Can you work these out from the model? Positions are in its coordinate system, mm. A direction names the side the tool comes from. Coordinates: 2 decimals unless noted, no trailing zeros. Write each loop counter-clockwise with the first axis right and the second up, starting at its lowest first coordinate (ties: lowest second). Pieces come first, ordered by that corner, then holes. Notation, with made-up numbers: (-5.75, 85.25) -> (11.25, 85.25) arc R20 ccw to (11.25, 104.25) -> close; hole circle Ø10 at (33.25, 3.25). An arc over 180 degrees is marked (long way). Use one line per item in the form item = value.
```python
from build123d import *

# Parameters (mm, degrees)
BOSS_EXTRUDE2_DEPTH       = 60
SKETCH4_W                 = 120
SKETCH4_H                 = 100
BOSS_EXTRUDE3_DEPTH       = 7.5
SKETCH5_W                 = 135
SKETCH5_H                 = 150
BOSS_EXTRUDE4_DEPTH       = 5
SKETCH6_W                 = 112.3
SKETCH6_H                 = 75
CUT_EXTRUDE2_DEPTH        = 75
F_10_CLEARANCE_HOLE1_D    = 4.7752
F_2_CLEARANCE_HOLE1_D     = 2.032
F_2_CLEARANCE_HOLE1_DEPTH = 6.35
F_2_CLEARANCE_HOLE1_TIP   = 0.610474389
SKETCH17_W                = 3
SKETCH17_H                = 3
CUT_EXTRUDE4_DEPTH        = 76
SKETCH18_R                = 2.5
CUT_EXTRUDE5_DEPTH        = 27
SKETCH19_R                = 1.5
CUT_EXTRUDE6_DEPTH        = 4


with BuildPart() as part:
    # Sketch3 → Boss-Extrude2 (new body, symmetric)
    with BuildSketch(Plane.XY):
        with BuildLine():
            Line((0, 0), (120, 0))
            Line((120, 0), (120, 100))
            Line((120, 100), (115, 100))
            ThreePointArc((115, 100), (54.85834395, 118.924191085), (0, 150))
            Line((0, 150), (0, 0))
        make_face()
    extrude(amount=BOSS_EXTRUDE2_DEPTH, both=True)

    # Sketch4 → Boss-Extrude3 (add)
    with BuildSketch(Plane.XY.offset(60)):
        with Locations((60, 50)):
            Rectangle(SKETCH4_W, SKETCH4_H)
    boss_extrude3 = extrude(amount=BOSS_EXTRUDE3_DEPTH)

    # Mirror1: Boss-Extrude3 across plane
    add(boss_extrude3.mirror(Plane.XY))

    # Sketch5 → Boss-Extrude4 (add)
    with BuildSketch(Plane.ZY):
        with Locations((0, 75)):
            Rectangle(SKETCH5_W, SKETCH5_H)
    extrude(amount=BOSS_EXTRUDE4_DEPTH)

    # Sketch6 → Cut-Extrude2 (cut)
    with BuildSketch(Plane.XZ):
        with Locations((51.15, 0)):
            Rectangle(SKETCH6_W, SKETCH6_H)
    extrude(amount=-CUT_EXTRUDE2_DEPTH, mode=Mode.SUBTRACT)

    # #10 Clearance Hole1 (through all)
    with Locations(Plane.ZY.offset(-107.3)):
        with Locations((0, 55), (0, 20)):
            Hole(F_10_CLEARANCE_HOLE1_D / 2)

    # #2 Clearance Hole1
    with Locations(Plane(origin=(0, 75, 0), x_dir=(-1, 0, 0), z_dir=(0, -1, 0))):
        with Locations((-20, 18.5), (-72, -14.25), (-72, 13.75), (-21.143, -29.5)):
            Hole(F_2_CLEARANCE_HOLE1_D / 2, depth=F_2_CLEARANCE_HOLE1_DEPTH)
            with Locations((0, 0, -(F_2_CLEARANCE_HOLE1_DEPTH + F_2_CLEARANCE_HOLE1_TIP / 2))):  # 118° drill point
                Cone(0, F_2_CLEARANCE_HOLE1_D / 2, F_2_CLEARANCE_HOLE1_TIP, mode=Mode.SUBTRACT)

    # Sketch15 → #10 Clearance Hole2 (revolve, cut)
    with BuildSketch(Plane(origin=(15, 115, 60), x_dir=(0, -1, 0), z_dir=(1, 0, 0))):
        Polygon((0, 0), (0, 26.849876674), (2.413, 25.4), (2.413, 0), align=None)
    f_10_clearance_hole2 = revolve(axis=Axis((15, 115, 66.35), (0, 0, -1)), mode=Mode.SUBTRACT)

    # Mirror2: #10 Clearance Hole2 across plane
    add(f_10_clearance_hole2.mirror(Plane.XY), mode=Mode.SUBTRACT)

    # Sketch17 → Cut-Extrude4 (cut, through all)
    with BuildSketch(Plane.XZ.offset(-75)):
        with Locations((4.5, 0)):
            Rectangle(SKETCH17_W, SKETCH17_H)
    extrude(amount=-CUT_EXTRUDE4_DEPTH, mode=Mode.SUBTRACT)

    # Sketch18 → Cut-Extrude5 (cut)
    with BuildSketch(Plane(origin=(0, 0, 37.5), x_dir=(-1, 0, 0), z_dir=(0, 0, -1))):
        with Locations((-67.5, 30)):
            Circle(SKETCH18_R)
        with Locations((-57.5, 30)):
            Circle(SKETCH18_R)
        with Locations((-47.5, 30)):
            Circle(SKETCH18_R)
    extrude(amount=-CUT_EXTRUDE5_DEPTH, mode=Mode.SUBTRACT)

    # Sketch19 → Cut-Extrude6 (cut, through all)
    with BuildSketch(Plane(origin=(0, 0, 64.5), x_dir=(-1, 0, 0), z_dir=(0, 0, -1))):
        with Locations((-67.5, 30)):
            Circle(SKETCH19_R)
        with Locations((-57.5, 30)):
            Circle(SKETCH19_R)
        with Locations((-47.5, 30)):
            Circle(SKETCH19_R)
    extrude(amount=-CUT_EXTRUDE6_DEPTH, mode=Mode.SUBTRACT)


solid = part.part
```
Q1. Suppose I cut it at B-B (z = -50). Write out the boundary of the cut face in (x, y).
Return value:
outline = (-5, 0) -> (120, 0) -> (120, 100) -> (115, 100) arc R300 cw to (0, 150) -> (-5, 150) -> close; hole circle Ø4.83 at (15, 115)
Q2. Suppose I cut it at D-D (x = 96.5). Write out the boundary of the cut face in (y, z).
Return value:
outline = (0, -67.5) -> (100, -67.5) -> (100, -60) -> (104.36, -60) -> (104.36, 60) -> (100, 60) -> (100, 67.5) -> (0, 67.5) -> (0, 37.5) -> (75, 37.5) -> (75, -37.5) -> (0, -37.5) -> close
Q3. If I drill on line 1 (Z direction, x = 92, y = 48); line 2 (X direction, y = 62.5, z = 28.5); line 3 (Y direction, x = 67.5, z = 66.05), over which ranges is the centre line in solid material (lowest first)? Write a range as from..to.
Return value:
line_1 = -67.5..-37.5, 37.5..67.5
line_2 = 107.3..120
line_3 = 0..28.5, 31.5..100
Q4. Suppose I cut it at A-A (z = -27). Write out the boundary of the cut face in (x, y), then the cut area to 3 significant figures.
Return value:
outline = (-5, 75) -> (107.3, 75) -> (107.3, 0) -> (120, 0) -> (120, 100) -> (115, 100) arc R300 cw to (0, 150) -> (-5, 150) -> close
area = 6,650 mm2
Q5. Suppose I cut it at C-C (y = 125). Write out the boundary of the cut face in (x, z).
Return value:
outline = (-5, -67.5) -> (0, -67.5) -> (0, -60) -> (41.76, -60) -> (41.76, 60) -> (0, 60) -> (0, 67.5) -> (-5, 67.5) -> close; hole (3, -1.5) -> (6, -1.5) -> (6, 1.5) -> (3, 1.5) -> close
Q6. For faces 1 (the flat face through (66, 29, 64.5)), 2 (the flat face through (31, 114, 60)), 3 (the flat face through (50, 75, 1)), which set-ups out of +Z, -Z, +X, -X, +Y, -Y let a thin tool reach every point of the face, with its end or its side?
Return value:
face_1 = none
face_2 = +Z, +X, +Y
face_3 = -X, -Y
Q7. Will these pins go through, and if not, where does the flat tip stop? pin 1 (12 mm diameter, centred on x = 46.5, z = -14.5, fed in from -Y); pin 2 (4 mm diameter, centred on x = 15, y = 115, fed in from +Z); pin 3 (1.5 mm diameter, centred on y = 121, z = -5.5, fed in from +X); pin 4 (4.5 mm diameter, centred on y = 55, z = 0, fed in from -X).
Return value:
pin_1 = 75
pin_2 = 34.35
pin_3 = 51.85
pin_4 = through
Q8. Thinking about a two-plate mould opening in Y: for faces 4 (the cylindrical face through (56, 32, 51)), 5 (the flat face through (50, 37, -37.5)), 6 (the cylindrical face through (55.67, 118.573, 0.84)), which applies, released by +Y, released by -Y, zero draft, split by the parting line, or undercut?
Return value:
face_4 = undercut
face_5 = zero draft
face_6 = released by +Y
